from build123d import *

# Parameters (mm, degrees)
SKETCH1_W        = 50
SKETCH1_H        = 50
SKETCH1_R        = 1.5
SUPPORT_DEPTH    = 8
NORTH_START      = -25
SKETCH2_W        = 20
SKETCH2_H        = 5
NORTH_CUT_DEPTH  = 4
EAST_START       = 25
SKETCH3_W        = 20
SKETCH3_H        = 5
EAST_DOWEL_DEPTH = 4


with BuildPart() as part:
    # Sketch1 → Support (new body)
    with BuildSketch(Plane(origin=(0, 0, 0), x_dir=(1, 0, 0), z_dir=(0, 1, 0))):
        Rectangle(SKETCH1_W, SKETCH1_H)
        with Locations(Location((-21, -21, 0), (0, 0, 270))):
            Circle(SKETCH1_R, mode=Mode.SUBTRACT)
        with Locations(Location((21, -21, 0), (0, 0, 270))):
            Circle(SKETCH1_R, mode=Mode.SUBTRACT)
        with BuildLine():
            Line((-13.031373033, 17.5), (17.5, 17.5))
            Line((17.5, 17.5), (17.5, -17.5))
            Line((17.5, -17.5), (-17.5, -17.5))
            Line((-17.5, -17.5), (-17.5, 13.031373033))
            ThreePointArc((-17.5, 13.031373033), (-20, 14.354248689), (-21, 17))
            Line((-21, 17), (-22.130136986, 20.01369863))
            ThreePointArc((-22.130136986, 20.01369863), (-22.060660172, 22.060660172), (-20.01369863, 22.130136986))
            Line((-20.01369863, 22.130136986), (-17, 21))
            ThreePointArc((-17, 21), (-14.354248689, 20), (-13.031373033, 17.5))
        make_face(mode=Mode.SUBTRACT)
        with Locations(Location((21, 21, 0), (0, 0, 270))):
            Circle(SKETCH1_R, mode=Mode.SUBTRACT)
    extrude(amount=SUPPORT_DEPTH)

    # Sketch2 → North Cut (cut)
    with BuildSketch(Plane.XY.offset(NORTH_START)):
        with Locations((0, 4)):
            Rectangle(SKETCH2_W, SKETCH2_H)
    extrude(amount=NORTH_CUT_DEPTH, mode=Mode.SUBTRACT)

    # Sketch3 → East Dowel (add)
    with BuildSketch(Plane(origin=(0, 0, 0), x_dir=(0, 0, -1), z_dir=(1, 0, 0)).offset(EAST_START)):
        with Locations((0, 4)):
            Rectangle(SKETCH3_W, SKETCH3_H)
    extrude(amount=EAST_DOWEL_DEPTH)


solid = part.part
Here's how the part is built. I have some questions about the finished solid (model axes, mm). A direction names the side the tool comes from. Give positions to 0.01 mm unless a question says otherwise; leave off trailing zeros. Order: outer loops, then holes, each group sorted by start corner. A loop starts at its lowest first (then second) coordinate and runs counter-clockwise, first axis right, second up. Notation, with made-up numbers: M 27,-12 L 66,-12 A21 ccw 66,0 Z; hole C 84,5.5 d10. An arc over 180 degrees is marked long. Answer as a JSON object with one key per item and string values. Group by question number.
1) Suppose I cut it at A-A, the plane z = 6. Write out the boundary of the cut face in (x, y).
2) We'd pull the mould along X, two halves only. Please class faces 6 (the cylindrical face through (22.01, 3.94, -22.11)), 7 (the flat face through (0, 4, 25)): pulls with the +X half, pulls with the -X half, needs draft (parallel to the pull), parting line crosses it, or undercut.
3) Suppose I cut it at C-C, the plane x = 21. Write out the boundary of the cut face in (y, z), plus the area to 3 significant figures.
4) I'm going to push flat-ended pins straight in: pin 1 Ø1.2 at (x, z) = (27, -3) entering from +Y; pin 2 Ø2.5 at (x, y) = (4.5, 4) entering from -Z; pin 3 Ø2.5 at (x, z) = (21, -21) entering from -Y; pin 4 Ø2 at (x, z) = (27, 2) entering from -Y. Where does each tip first touch, or does it pass through?
5) Suppose I cut it at D-D, the plane y = 5. Write out the boundary of the cut face in (x, z), plus the area to 3 significant figures.
6) On a 3-axis mill with a long thin cutter (end or side, diameter ignored), from which of +Z, -Z, +X, -X, +Y, -Y can I reach the whole of each face in a straight line? I mean faces 1 (the flat face through (10, 4, -23)), 2 (the flat face through (-23, 8, 0)), 3 (the flat face through (27, 1.5, 0)), 4 (the flat face through (-21.56, 3.94, -18.49)), 5 (the flat face through (27, 4, -10)). Say none if no direction works.
7) Please list where these lines run through material, in increasing order: L1, parallel to X at y = 4.5, z = 21; L2, parallel to Z at x = -7, y = 5; L3, parallel to Z at x = -5, y = 0.5. Write a range as [from, to].
8) Suppose I cut it at B-B, the plane x = -4. Write out the boundary of the cut face in (y, z).
Results found:
{
 "1": {"outline": "M -25,0 L -17.5,0 L -17.5,8 L -25,8 Z; M 17.5,0 L 25,0 L 25,1.5 L 29,1.5 L 29,6.5 L 25,6.5 L 25,8 L 17.5,8 Z"},
 "2": {"face 6": "undercut", "face 7": "needs draft"},
 "3": {"outline": "M 0,-25 L 8,-25 L 8,-22.5 L 0,-22.5 Z; M 0,-19.5 L 8,-19.5 L 8,19.5 L 0,19.5 Z; M 0,22.5 L 8,22.5 L 8,25 L 0,25 Z", "area": "352 mm²"},
 "4": {"pin 1": "y = 6.5", "pin 2": "z = -21", "pin 3": "through", "pin 4": "y = 1.5"},
 "5": {"outline": "M -25,-25 L -10,-25 L -10,-21 L 10,-21 L 10,-25 L 25,-25 L 25,-10 L 29,-10 L 29,10 L 25,10 L 25,25 L -25,25 Z; hole C -21,21 d3; hole M -22.13,-20.01 A1.5 ccw -20.01,-22.13 L -17,-21 A4 ccw -13.03,-17.5 L 17.5,-17.5 L 17.5,17.5 L -17.5,17.5 L -17.5,-13.03 A4 ccw -21,-17 Z; hole C 21,-21 d3; hole C 21,21 d3", "area": "1,210 mm²"},
 "6": {"face 1": "-Z", "face 2": "+Z, -Z, +X, -X, +Y", "face 3": "+Z, -Z, +X, -Y", "face 4": "+Y, -Y", "face 5": "-Z, +X, +Y, -Y"},
 "7": {"L1": "[-25, -22.5], [-19.5, 19.5], [22.5, 25]", "L2": "[-21, -17.5], [17.5, 25]", "L3": "[-25, -17.5], [17.5, 25]"},
 "8": {"outline": "M 0,-25 L 1.5,-25 L 1.5,-21 L 6.5,-21 L 6.5,-25 L 8,-25 L 8,-17.5 L 0,-17.5 Z; M 0,17.5 L 8,17.5 L 8,25 L 0,25 Z"}
}
